Can you work these out from the drawing? Everything is in mm from the part's minimum corner. A direction names the side the tool comes from. Coordinates: 2 decimals unless noted, no trailing zeros. Write each loop counter-clockwise with the first axis right and the second up, starting at its lowest first coordinate (ties: lowest second). Pieces come first, ordered by that corner, then holes. Notation, with made-up numbers: M 57.25,42.25 L 95.25,42.25 A18 ccw 95.25,72.25 Z; hole C -39.75,54.5 d10. An arc over 180 degrees is marked long. Write item = value, one per line.
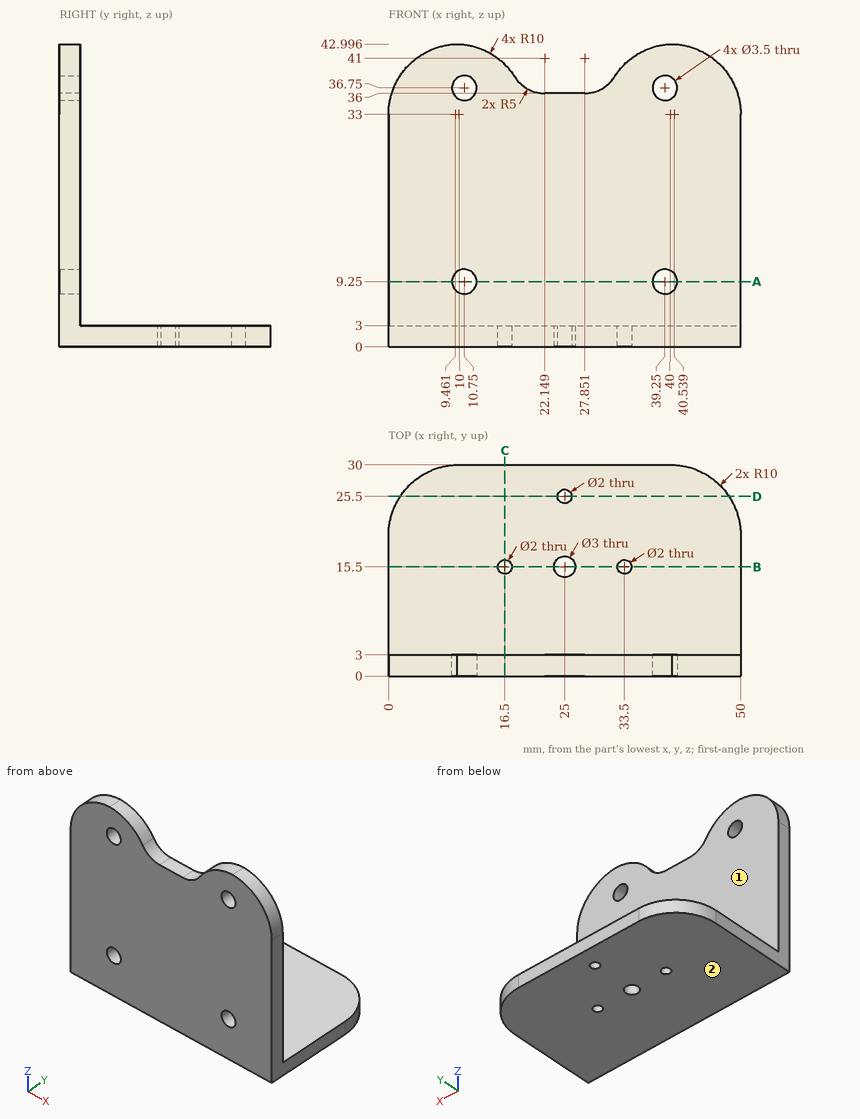
Item 1: Imagine slicing it at A-A (z = 9.25). Write out the boundary of the cut face in (x, y), and give its area (3 significant figures).
Numbers:
outline = M 0,0 L 9,0 L 9,3 L 0,3 Z; M 12.5,0 L 37.5,0 L 37.5,3 L 12.5,3 Z; M 41,0 L 50,0 L 50,3 L 41,3 Z
area = 129 mm²
Item 2: Imagine slicing it at D-D (y = 25.5). Write out the boundary of the cut face in (x, z), and give its area (3 significant figures).
Numbers:
outline = M 1.65,0 L 24,0 L 24,3 L 1.65,3 Z; M 26,0 L 48.35,0 L 48.35,3 L 26,3 Z
area = 134 mm²
Item 3: Imagine slicing it at B-B (y = 15.5). Write out the boundary of the cut face in (x, z).
Numbers:
outline = M 0,0 L 15.5,0 L 15.5,3 L 0,3 Z; M 17.5,0 L 23.5,0 L 23.5,3 L 17.5,3 Z; M 26.5,0 L 32.5,0 L 32.5,3 L 26.5,3 Z; M 34.5,0 L 50,0 L 50,3 L 34.5,3 Z
Item 4: For the marked faces 1 and 2, which set-ups out of +Z, -Z, +X, -X, +Y, -Y let a thin tool reach every point of the face, with its end or its side?
Numbers:
face_1 = +Z, +X, -X, +Y
face_2 = -Z, +X, -X, +Y, -Y
Item 5: If I drill on line 1 along Y through (x, z) = (25, 1.4); line 2 along X through (y, z) = (15.5, 1.75); line 3 along Y through (x, z) = (16, 24), over which ranges is the centre line in solid material (lowest first)?
Numbers:
line_1 = 0 to 14, 17 to 24.5, 26.5 to 30
line_2 = 0 to 15.5, 17.5 to 23.5, 26.5 to 32.5, 34.5 to 50
line_3 = 0 to 3
Item 6: I'm going to push flat-ended pins straight in: P1, Ø1.8, axis at x = 25, y = 15.5, coming from the -Z side; P2, Ø3, axis at x = 18, y = 18.5, coming from the -Z side; P3, Ø13.5, axis at x = 21.5, y = 23, coming from the +Z side; P4, Ø0.9, axis at x = 24.5, y = 1, coming from the +Z side. Where does each tip first touch, or does it pass through?
Numbers:
P1 = through
P2 = 0
P3 = 3
P4 = 36
Item 7: Imagine slicing it at C-C (x = 16.5). Write out the boundary of the cut face in (y, z).
Numbers:
outline = M 0,0 L 14.5,0 L 14.5,3 L 3,3 L 3,40.1 L 0,40.1 Z; M 16.5,0 L 30,0 L 30,3 L 16.5,3 Z
